```python
from build123d import *

# Parameters (mm, degrees)
ARM_BASE_SKETCH_W                  = 12
ARM_BASE_SKETCH_H                  = 115
ARM_BASE_EXTRUDE_DEPTH             = 5
SCREW_BASES_SKETCH_R               = 6
SCREW_BASES_EXTRUDE_DEPTH          = 8.25
POWER_SUPPLY_MOUNTING_SLOT_DEPTH   = 8.25
POWER_SUPPLY_MOUNTING_SLOT_2_DEPTH = 3.1
NO_6_MOUNTING_SCREWS_D             = 3.7973
NO_6_MOUNTING_SCREWS_CSINK_D       = 10.563733
NO_6_MOUNTING_SCREWS_CSINK_ANGLE   = 82


# Read off the part's stored shape, not the designer's step: Power Supply Mounting Slot
with BuildPart() as part:
    # Arm Base Sketch → Arm Base Extrude (new body)
    with BuildSketch(Plane(origin=(0, 0, 0), x_dir=(1, 0, 0), z_dir=(0, 1, 0))):
        with Locations((0, 57.5)):
            Rectangle(ARM_BASE_SKETCH_W, ARM_BASE_SKETCH_H)
    extrude(amount=ARM_BASE_EXTRUDE_DEPTH)

    # Screw Bases Sketch → Screw Bases Extrude (add)
    with BuildSketch(Plane.XZ):
        with Locations(Location((0, -115, 0), (0, 0, 270))):
            Circle(SCREW_BASES_SKETCH_R)
        with BuildLine():
            Line((-8, -81), (-8, -69))
            ThreePointArc((-8, -69), (0, -61), (8, -69))
            Line((8, -69), (8, -81))
            ThreePointArc((8, -81), (0, -89), (-8, -81))
        make_face()
    extrude(amount=-SCREW_BASES_EXTRUDE_DEPTH)

    # Power Supply Mounting Slot outline → Power Supply Mounting Slot (cut)
    with BuildSketch(Plane(origin=(0, 0, 0), x_dir=(1, 0, 0), z_dir=(0, 1, 0))):
        with BuildLine():
            ThreePointArc((-2.25, 71.25), (0, 69), (2.25, 71.25))
            Line((2.25, 71.25), (2.25, 78.75))
            ThreePointArc((2.25, 78.75), (0, 81), (-2.25, 78.75))
            Line((-2.25, 78.75), (-2.25, 71.25))
        make_face()
    extrude(amount=POWER_SUPPLY_MOUNTING_SLOT_DEPTH, mode=Mode.SUBTRACT)

    # Power Supply Mounting Slot 2 outline → Power Supply Mounting Slot 2 (cut)
    with BuildSketch(Plane(origin=(0, 0, 0), x_dir=(1, 0, 0), z_dir=(0, 1, 0))):
        with BuildLine():
            ThreePointArc((-4.5, 71.25), (0, 66.75), (4.5, 71.25))
            Line((4.5, 71.25), (4.5, 78.75))
            ThreePointArc((4.5, 78.75), (0, 83.25), (-4.5, 78.75))
            Line((-4.5, 78.75), (-4.5, 71.25))
        make_face()
        with BuildLine():
            Line((2.25, 78.75), (2.25, 71.25))
            ThreePointArc((2.25, 71.25), (0, 69), (-2.25, 71.25))
            Line((-2.25, 71.25), (-2.25, 78.75))
            ThreePointArc((-2.25, 78.75), (0, 81), (2.25, 78.75))
        make_face(mode=Mode.SUBTRACT)
    extrude(amount=POWER_SUPPLY_MOUNTING_SLOT_2_DEPTH, mode=Mode.SUBTRACT)

    # No. 6 Mounting Screws (through all)
    with Locations(Plane(origin=(0, 8.25, 0), x_dir=(1, 0, 0), z_dir=(0, 1, 0))):
        with Locations((0, 115)):
            CounterSinkHole(NO_6_MOUNTING_SCREWS_D / 2, NO_6_MOUNTING_SCREWS_CSINK_D / 2, counter_sink_angle=NO_6_MOUNTING_SCREWS_CSINK_ANGLE)

    # Mirror 2: part across plane


with BuildPart() as part_1:
    add(part.part)
    add(part.part.mirror(Plane(origin=(6, 5, 0), x_dir=(1, 0, 0), z_dir=(0, 0, -1))))


solid = part_1.part
```
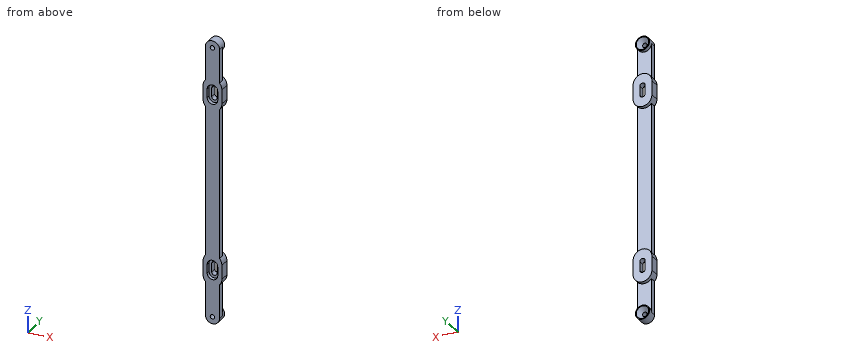
Source: CAD feature listing. Evaluate the final solid. Frame: model axes, mm. Coordinates: 2 decimals unless noted, no trailing zeros. Order: outer loops, then holes, each group sorted by start corner. A loop starts at its lowest first (then second) coordinate and runs counter-clockwise, first axis right, second up. Notation, with made-up numbers: M 77.25,-27 L 114.25,-27 A12 ccw 114.25,-15 Z; hole C 41.5,28.25 d4. An arc over 180 degrees is marked long. Write each question's results on one line, items separated by ' | '. Start each with the question number.
1) Line query: line 1 (Z direction, x = 0, y = 2.65); line 2 (Z direction, x = 0, y = 3.3); line 3 (X direction, y = 2.95, z = -115). Output: solid intervals per line, ascending. Write a range as from..to.
2) Section query A-A (z = 76). Return the cut outline in (x, y).
3) Contact query for flat-ended pins moving along their axis: pin 1 Ø2 at (y, z) = (2, 44.5) entering from -X; pin 2 Ø6 at (x, z) = (-1, 104.5) entering from +Y; pin 3 Ø2 at (y, z) = (4, 55) entering from +X. Output: stop coordinate, or through.
4) Section query B-B (y = 7). Return the cut outline in (x, z).
Answers:
1) line 1: z = -121..-116.9, -113.1..-83.25, -66.75..66.75, 83.25..113.1, 116.9..121 | line 2: z = -121..-116.9, -113.1..-81, -69..69, 81..113.1, 116.9..121 | line 3: x = -6..-1.9, 1.9..6
2) outline: M -8,0 L -4.5,0 L -4.5,3.1 L -2.25,3.1 L -2.25,8.25 L -8,8.25 Z; M 2.25,3.1 L 4.5,3.1 L 4.5,0 L 8,0 L 8,8.25 L 2.25,8.25 Z
3) pin 1: stops at x = -6 | pin 2: stops at y = 5 | pin 3: stops at x = 6
4) outline: M -8,-81 A8 ccw 8,-81 L 8,-69 A8 ccw -8,-69 Z; M -8,69 A8 ccw 8,69 L 8,81 A8 ccw -8,81 Z; C 0,-115 d12; C 0,115 d12; hole C 0,-115 d8.39; hole C 0,115 d8.39; hole M -2.25,-78.75 A2.25 ccw 2.25,-78.75 L 2.25,-71.25 A2.25 ccw -2.25,-71.25 Z; hole M -2.25,71.25 A2.25 ccw 2.25,71.25 L 2.25,78.75 A2.25 ccw -2.25,78.75 Z
